from build123d import *

# Parameters (mm, degrees)
SKETCH1_R           = 6.75
SKETCH1_W           = 15
SKETCH1_H           = 15
BOSS_EXTRUDE1_DEPTH = 12
CUT_EXTRUDE1_REACH  = 64.336
SKETCH2_R           = 1.75
FILLET1_R           = 3
SKETCH3_R           = 11.25
CUT_EXTRUDE2_DEPTH  = 9


with BuildPart() as part:
    # Sketch1 → Boss-Extrude1 (new body)
    with BuildSketch(Plane.XY):
        with BuildLine():
            Line((-18.868931919, 14.90275594), (3.131068081, 14.90275594))
            Line((3.131068081, 14.90275594), (3.131068081, -7.09724406))
            Line((3.131068081, -7.09724406), (-18.868931919, -7.09724406))
            Line((-18.868931919, -7.09724406), (-18.868931919, -1.09724406))
            Line((-18.868931919, -1.09724406), (-26.226796295, -1.09724406))
            ThreePointArc((-26.226796295, -1.09724406), (-55.368931919, 3.90275594), (-26.226796295, 8.90275594))
            Line((-26.226796295, 8.90275594), (-18.868931919, 8.90275594))
            Line((-18.868931919, 8.90275594), (-18.868931919, 14.90275594))
        make_face()
        with Locations((-40.368931919, 3.90275594)):
            Circle(SKETCH1_R, mode=Mode.SUBTRACT)
        with Locations((-7.868931919, 3.90275594)):
            Rectangle(SKETCH1_W, SKETCH1_H, mode=Mode.SUBTRACT)
    extrude(amount=BOSS_EXTRUDE1_DEPTH)

    # Cut-Extrude1: up to this face of the body (flat: up to its plane)
    cut_extrude1_end = Plane(part.part.faces().sort_by_distance((-7.868931919, 14.90275594, 6))[0])
    # Sketch2 → Cut-Extrude1 (cut, up to the picked face)
    with BuildSketch(Plane.XZ.offset(7.09724406), mode=Mode.PRIVATE) as cut_extrude1_sk1:
        with Locations(Location((-7.868931919, 6, 0), (0, 0, 270))):
            Circle(SKETCH2_R)
    cut_extrude1_tool1 = split(extrude(cut_extrude1_sk1.sketch, amount=-CUT_EXTRUDE1_REACH, mode=Mode.PRIVATE), bisect_by=cut_extrude1_end, keep=Keep.BOTH, mode=Mode.PRIVATE)
    add(cut_extrude1_tool1.solids().sort_by(Axis((-7.868932, -7.097244, 6), (0, 1, 0)))[0], mode=Mode.SUBTRACT)

    # Fillet1
    fillet1_edges = [part.edges().sort_by_distance(p)[0] for p in [
        (-18.868931919, -1.09724406, 6),
        (-26.226796295, -1.09724406, 6),
        (-26.226796295, 8.90275594, 6),
        (-18.868931919, 8.90275594, 6),
    ]]
    fillet(fillet1_edges, radius=FILLET1_R)

    # Sketch3 → Cut-Extrude2 (cut)
    with BuildSketch(Plane.XY.offset(12)):
        with Locations((-40.368931919, 3.90275594)):
            Circle(SKETCH3_R)
    extrude(amount=-CUT_EXTRUDE2_DEPTH, mode=Mode.SUBTRACT)


solid = part.part
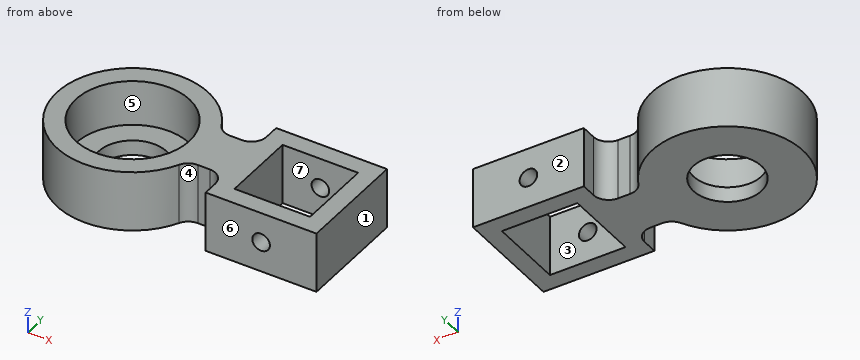
Input: part model. Units: mm. Frame: model coordinates. Face numbers are marked on the shaded views. A direction names the side the tool comes from. Give positions to 0.01 mm unless a question says otherwise; leave off trailing zeros. Loops run counter-clockwise (first coordinate to the right, second up) from the corner with the lowest first, then second, coordinate; pieces in that order, holes last. Notation, with made-up numbers: (9, -30) - (47, -30) arc R24 cw to (47, -19) - close; hole circle Ø3 at (4.5, 21). An arc over 180 degrees is marked (long way). Use CSV: the item, a comma, the result in double quotes. Start each with the question number.
Item 1: Line query: line 1 (X direction, y = 4, z = 10.5); line 2 (Y direction, x = -8, z = 8); line 3 (X direction, y = -5.5, z = 6). Output: solid intervals per line, ascending.
Item 2: Section B-B on y = 1. Return loops of the section in (x, z).
Item 3: Section C-C on x = -12. Return loops of the section in (y, z).
Item 4: Section A-A on z = 6.75. Return loops of the section in (x, y).
Item 5: Mould query, pull axis X, two halves, no side actions, for the marked faces 1, 2 and 3. Classes: pulls with the +X half, pulls with the -X half, needs draft (parallel to the pull), parting line crosses it, or undercut.
Item 6: Contact query for flat-ended pins moving along their axis: P1, Ø1.5, axis at x = -13, z = 5, coming from the -Y side; P2, Ø2, axis at x = -7.87, z = 6, coming from the -Y side; P3, Ø1.5, axis at y = -5, z = 3, coming from the -X side; P4, Ø6, axis at x = -4.5, z = 5.5, coming from the +Y side. Output: stop coordinate, or through.
Item 7: Reachability of the marked faces 4, 5, 6 and 7 from +Z, -Z, +X, -X, +Y, -Y: full face, straight path, thin tool, end or side. Return the list, or none.
Item 8: Section D-D on z = 10. Return loops of the section in (x, y).
Ans:
1,line 1,"x = -55.37 to -51.62, -29.12 to -15.37, -0.37 to 3.13"
1,line 2,"y = -7.1 to -3.6, 11.4 to 14.9"
1,line 3,"x = -52.06 to -46.55, -34.19 to -28.68, -18.87 to -9.62, -6.12 to 3.13"
2,outline,"(-55.09, 0) - (-46.46, 0) - (-46.46, 3) - (-51.24, 3) - (-51.24, 12) - (-55.09, 12) - close; (-34.27, 0) - (-15.37, 0) - (-15.37, 12) - (-29.5, 12) - (-29.5, 3) - (-34.27, 3) - close; (-0.37, 0) - (3.13, 0) - (3.13, 12) - (-0.37, 12) - close"
3,outline,"(-7.1, 0) - (-3.6, 0) - (-3.6, 12) - (-7.1, 12) - close; (11.4, 0) - (14.9, 0) - (14.9, 12) - (11.4, 12) - close"
4,outline,"(-26.93, -2.76) arc R3 cw to (-24.24, -1.1) - (-21.87, -1.1) arc R3 cw to (-18.87, -4.1) - (-18.87, -7.1) - (-9.45, -7.1) - (-9.45, -3.6) - (-15.37, -3.6) - (-15.37, 11.4) - (-9.45, 11.4) - (-9.45, 14.9) - (-18.87, 14.9) - (-18.87, 11.9) arc R3 cw to (-21.87, 8.9) - (-24.24, 8.9) arc R3 cw to (-26.93, 10.57) arc R15 ccw (long way) to start; (-6.29, -7.1) - (3.13, -7.1) - (3.13, 14.9) - (-6.29, 14.9) - (-6.29, 11.4) - (-0.37, 11.4) - (-0.37, -3.6) - (-6.29, -3.6) - close; hole circle Ø22.5 at (-40.37, 3.9)"
5,face 1,"pulls with the +X half"
5,face 2,"needs draft"
5,face 3,"undercut"
6,P1,"stops at y = -7.1"
6,P2,"passes through"
6,P3,"stops at x = -52.96"
6,P4,"stops at y = 14.9"
7,face 4,"+Z, -Z, -Y"
7,face 5,"+Z"
7,face 6,"+Z, -Z, +X, -Y"
7,face 7,"+Z, -Z"
8,outline,"(-26.93, -2.76) arc R3 cw to (-24.24, -1.1) - (-21.87, -1.1) arc R3 cw to (-18.87, -4.1) - (-18.87, -7.1) - (3.13, -7.1) - (3.13, 14.9) - (-18.87, 14.9) - (-18.87, 11.9) arc R3 cw to (-21.87, 8.9) - (-24.24, 8.9) arc R3 cw to (-26.93, 10.57) arc R15 ccw (long way) to start; hole circle Ø22.5 at (-40.37, 3.9); hole (-15.37, -3.6) - (-0.37, -3.6) - (-0.37, 11.4) - (-15.37, 11.4) - close"
